Could you check a few things on this model? Use its own coordinates, in mm. A direction names the side the tool comes from. Round coordinates to 2 decimals unless told otherwise and drop trailing zeros. Write each loop counter-clockwise with the first axis right and the second up, starting at its lowest first coordinate (ties: lowest second). Pieces come first, ordered by that corner, then holes. Notation, with made-up numbers: M 47,1.5 L 82,1.5 A13 ccw 82,20.5 Z; hole C 54,34 d3. An arc over 180 degrees is marked long. One line per question, with ' | ' between items. Start each with the question number.
```python
from build123d import *

# Parameters (mm, degrees)
BOSS_EXTRUDE1_DEPTH = 14.4
SKETCH2_R           = 11.81943886
SKETCH2_R_2         = 1
CUT_EXTRUDE1_DEPTH  = 0.8
SKETCH3_W           = 6.542631095
SKETCH3_H           = 5.500743834
SKETCH3_W_2         = 5.841537105
CUT_EXTRUDE2_DEPTH  = 12
CUT_EXTRUDE3_DEPTH  = 24.277671705
CUT_EXTRUDE4_DEPTH  = 28.520356102
SKETCH6_R           = 9.65525988
SKETCH6_R_2         = 0.23
CUT_EXTRUDE5_DEPTH  = 3


with BuildPart() as part:
    # Sketch1 → Boss-Extrude1 (new body)
    with BuildSketch(Plane(origin=(0, 0, 0), x_dir=(1, 0, 0), z_dir=(0, 1, 0))):
        with BuildLine():
            Line((-10.8, 11.118003418), (-10.8, 8.428003418))
            Line((-10.8, 8.428003418), (-6.8, 8.428003418))
            Line((-6.8, 8.428003418), (-6.8, 7.258003418))
            Line((-6.8, 7.258003418), (6.8, 7.258003418))
            Line((6.8, 7.258003418), (6.8, 8.428003418))
            Line((6.8, 8.428003418), (10.8, 8.428003418))
            Line((10.8, 8.428003418), (10.8, 11.118003418))
            ThreePointArc((10.8, 11.118003418), (0, 15.5), (-10.8, 11.118003418))
        make_face()
    extrude(amount=BOSS_EXTRUDE1_DEPTH)

    # Sketch2 → Cut-Extrude1 (cut)
    with BuildSketch(Plane.XZ):
        with Locations((0, -10.948003418)):
            Circle(SKETCH2_R)
        with Locations(Location((-6.4, -10.948003418, 0), (0, 0, 270))):
            Circle(SKETCH2_R_2, mode=Mode.SUBTRACT)
        with Locations(Location((6.4, -10.948003418, 0), (0, 0, 270))):
            Circle(SKETCH2_R_2, mode=Mode.SUBTRACT)
    extrude(amount=-CUT_EXTRUDE1_DEPTH, mode=Mode.SUBTRACT)

    # Sketch3 → Cut-Extrude2 (cut)
    with BuildSketch(Plane(origin=(0, 14.4, 0), x_dir=(1, 0, 0), z_dir=(0, 1, 0))):
        with Locations((-10.071315548, 11.178375335)):
            Rectangle(SKETCH3_W, SKETCH3_H)
        with Locations((9.720768553, 11.178375335)):
            Rectangle(SKETCH3_W_2, SKETCH3_H)
    extrude(amount=-CUT_EXTRUDE2_DEPTH, mode=Mode.SUBTRACT)

    # Sketch4 → Cut-Extrude3 (cut, through all)
    with BuildSketch(Plane.XZ.offset(-0.8)):
        with BuildLine():
            Line((9.7, -11.118003418), (9.7, -12.089665008))
            Line((9.7, -12.089665008), (9.7, -13.215142829))
            Line((9.7, -13.215142829), (8.1, -13.215142829))
            Line((8.1, -13.215142829), (8.1, -11.118003418))
            ThreePointArc((8.1, -11.118003418), (8.9, -10.318003418), (9.7, -11.118003418))
        make_face()
        with BuildLine():
            Line((-8.1, -11.118003418), (-8.1, -13.215142829))
            Line((-8.1, -13.215142829), (-9.7, -13.215142829))
            Line((-9.7, -13.215142829), (-9.7, -11.118003418))
            ThreePointArc((-9.7, -11.118003418), (-8.9, -10.318003418), (-8.1, -11.118003418))
        make_face()
    extrude(amount=-CUT_EXTRUDE3_DEPTH, mode=Mode.SUBTRACT)

    # Sketch5 → Cut-Extrude4 (cut, through all)
    with BuildSketch(Plane.ZY.offset(6.8)):
        with BuildLine():
            Line((-12.628003418, 6.59), (-7.258003418, 6.59))
            Line((-7.258003418, 6.59), (-7.258003418, 4.81))
            Line((-7.258003418, 4.81), (-12.628003418, 4.81))
            ThreePointArc((-12.628003418, 4.81), (-13.518003418, 5.7), (-12.628003418, 6.59))
        make_face()
    extrude(amount=-CUT_EXTRUDE4_DEPTH, mode=Mode.SUBTRACT)

    # Sketch6 → Cut-Extrude5 (cut)
    with BuildSketch(Plane(origin=(0, 14.4, 0), x_dir=(1, 0, 0), z_dir=(0, 1, 0))):
        with Locations((0, 7.666269644)):
            Circle(SKETCH6_R)
        with Locations(Location((0, 7.666269644, 0), (0, 0, 270))):
            Circle(SKETCH6_R_2, mode=Mode.SUBTRACT)
        with Locations(Location((1.27, 7.666269644, 0), (0, 0, 270))):
            Circle(SKETCH6_R_2, mode=Mode.SUBTRACT)
        with Locations(Location((2.54, 7.666269644, 0), (0, 0, 270))):
            Circle(SKETCH6_R_2, mode=Mode.SUBTRACT)
        with Locations(Location((-1.27, 7.666269644, 0), (0, 0, 270))):
            Circle(SKETCH6_R_2, mode=Mode.SUBTRACT)
        with Locations(Location((-2.54, 7.666269644, 0), (0, 0, 270))):
            Circle(SKETCH6_R_2, mode=Mode.SUBTRACT)
    extrude(amount=-CUT_EXTRUDE5_DEPTH, mode=Mode.SUBTRACT)


solid = part.part
```
1. If we mould it in two halves opening along Y, with no side actions, what happens to faces 1 (the face through (0, 9, -7.258)), 2 (the face through (6, 0, -11)), 3 (the face through (0, 4.81, -10))? For each: released by +Y, released by -Y, zero draft, split by the parting line, or undercut.
2. Suppose I cut it at C-C (z = -10.75). Write out the boundary of the cut face in (x, y).
3. I'm going to push flat-ended pins straight in: P1, Ø1.2, axis at x = -9.5, z = -10.5, coming from the +Y side; P2, Ø1.3, axis at y = 1.5, z = -12, coming from the +X side; P3, Ø0.8, axis at x = 9, y = 1, coming from the +Z side; P4, Ø1.1, axis at y = 1.5, z = -11.5, coming from the +X side. Where does each tip first touch, or does it pass through?
4. Which directions (+Z, -Z, +X, -X, +Y, -Y) give clear straight access to the entire face, cutting with the end or side of a thin tool? Please do faces 4 (the face through (-8.1, 2, -12)), 5 (the face through (5.792, 0.394, -10.154)), 6 (the face through (-9, 2, -8.428)).
5. Suppose I cut it at B-B (z = -8.75). Write out the boundary of the cut face in (x, y).
6. I need wall thicknesses on line 1 along Y through (x, z) = (1.5, -8.5); line 2 along Y through (x, z) = (6.25, -11); line 3 along X through (y, z) = (11.25, -10.75). Which ranges of each line are inside material? Lowest first, please. Write a range as from..to.
7. Suppose I cut it at D-D (x = 0). Write out the boundary of the cut face in (y, z), and give its area (3 significant figures).
8. Suppose I cut it at A-A (y = 13.5). Write out the boundary of the cut face in (x, z).
Computed:
1) face 1: zero draft | face 2: released by -Y | face 3: undercut
2) outline: M -10.8,0.8 L -9.61,0.8 L -9.61,2.4 L -10.8,2.4 Z; M -8.19,0.8 L -7.38,0.8 L -7.38,0 L -5.42,0 L -5.42,0.8 L 5.42,0.8 L 5.42,0 L 7.38,0 L 7.38,0.8 L 8.19,0.8 L 8.19,2.4 L 6.8,2.4 L 6.8,4.81 L -6.8,4.81 L -6.8,2.4 L -8.19,2.4 Z; M -6.8,6.59 L 6.8,6.59 L 6.8,11.4 L -6.8,11.4 Z; M 9.61,0.8 L 10.8,0.8 L 10.8,2.4 L 9.61,2.4 Z
3) P1: stops at y = 2.4 | P2: stops at x = 10.56 | P3: stops at z = -8.43 | P4: stops at x = 10.8
4) face 4: -Z, +Y, -Y | face 5: -Y | face 6: +Z, -X, +Y, -Y
5) outline: M -10.8,0.8 L 10.8,0.8 L 10.8,2.4 L 6.8,2.4 L 6.8,4.81 L -6.8,4.81 L -6.8,2.4 L -10.8,2.4 Z; M -6.8,6.59 L 6.8,6.59 L 6.8,11.4 L -6.8,11.4 Z
6) line 1: y = 0.8..4.81, 6.59..11.4 | line 2: y = 0..4.81, 6.59..11.4 | line 3: x = -6.8..6.8
7) outline: M 0.8,-15.5 L 11.4,-15.5 L 11.4,-7.9 L 14.4,-7.9 L 14.4,-7.44 L 11.4,-7.44 L 11.4,-7.26 L 6.59,-7.26 L 6.59,-12.63 A0.89 cw 4.81,-12.63 L 4.81,-7.26 L 0.8,-7.26 Z | area: 77.9 mm²
8) outline: C -2.54,-7.67 d0.46; C -1.27,-7.67 d0.46; C 0,-7.67 d0.46; C 1.27,-7.67 d0.46; C 2.54,-7.67 d0.46
